Part model, mm, in its own coordinate system. A direction names the side the tool comes from. Round coordinates to 2 decimals unless told otherwise and drop trailing zeros. Write each loop counter-clockwise with the first axis right and the second up, starting at its lowest first coordinate (ties: lowest second). Pieces come first, ordered by that corner, then holes. Notation, with made-up numbers: M 21,0.25 L 61,0.25 A23 ccw 61,25.25 Z; hole C 36,-1 d2. An arc over 180 degrees is marked long. Use one line per item in the form item = value. Start each with the question number.
Item 1: Probe L1, parallel to X at y = 0, z = 15; L2, parallel to X at y = -1.5, z = 7.5; L3, parallel to Y at x = -19, z = 56. List the from-to ranges inside material, lowest first.
Item 2: Cut at A-A, the plane y = 0. Give the cut face in (x, z).
Item 3: Cut at D-D, the plane y = -5. Give the cut face in (x, z).
Item 4: Flat gauge pins, fed straight in: pin 1 Ø3 at (x, y) = (4, -20) entering from -Z; pin 2 Ø8 at (x, y) = (-16.46, 16.07) entering from +Z; pin 3 Ø1.5 at (x, z) = (5, 24.5) entering from -Y. Where does each tip first touch, or does it go through?
Item 5: Cut at B-B, the plane y = -14.5. Give the cut face in (x, z).
Item 6: Which spindle directions (+Z, -Z, +X, -X, +Y, -Y) get a long thin tool onto all of the face, cutting with end or side? Do faces 1 (the face through (0, 21, 56)), 2 (the face through (20.859, -21.297, 29.58)), 3 (the face through (-20, -2, 59)), 4 (the face through (0, -21, 52)), 5 (the face through (13.68, -18.2, 29.58)). Say none if no direction does.
Item 7: Cut at C-C, the plane z = 35.5. Give the cut face in (x, y), then the cut area to 3 significant figures.
Item 8: Mould opens along Z. For faces 6 (the face through (-28, 0, 30)), 7 (the face through (0, 21, 34)) say: +Z half, -Z half, draft (parallel to the pull), parting line (faces both ways), or undercut.
from build123d import *

# Parameters (mm, degrees)
SKETCH1_R               = 16
SKETCH1_R_2             = 3.5
SKETCH1_R_3             = 2
BOSS_EXTRUDE1_DEPTH     = 60
SKETCH2_R               = 18
SKETCH2_R_2             = 16
BOSS_EXTRUDE2_DEPTH     = 2
CUT_EXTRUDE1_DEPTH      = 2
SKETCH6_W               = 4
SKETCH6_H               = 24
LPATTERN1_COUNT         = 9
LPATTERN1_PITCH         = 6
MIRROR1_COPY_1_SKETCH_W = 4
MIRROR1_COPY_1_SKETCH_H = 24
MIRROR1_COPY_2_SKETCH_W = 4
MIRROR1_COPY_2_SKETCH_H = 24
MIRROR1_COPY_3_SKETCH_W = 4
MIRROR1_COPY_3_SKETCH_H = 24
MIRROR1_COPY_4_SKETCH_W = 4
MIRROR1_COPY_4_SKETCH_H = 24
MIRROR1_COPY_5_SKETCH_W = 4
MIRROR1_COPY_5_SKETCH_H = 24
MIRROR1_COPY_6_SKETCH_W = 4
MIRROR1_COPY_6_SKETCH_H = 24
MIRROR1_COPY_7_SKETCH_W = 4
MIRROR1_COPY_7_SKETCH_H = 24
MIRROR1_COPY_8_SKETCH_W = 4
MIRROR1_COPY_8_SKETCH_H = 24


with BuildPart() as part:
    # Sketch1 → Boss-Extrude1 (new body)
    with BuildSketch(Plane.XY):
        with BuildLine():
            Line((-24, 22.5), (18, 22.5))
            ThreePointArc((18, 22.5), (20.828427125, 21.328427125), (22, 18.5))
            Line((22, 18.5), (22, -18.5))
            ThreePointArc((22, -18.5), (20.828427125, -21.328427125), (18, -22.5))
            Line((18, -22.5), (-24, -22.5))
            ThreePointArc((-24, -22.5), (-26.828427125, -21.328427125), (-28, -18.5))
            Line((-28, -18.5), (-28, 18.5))
            ThreePointArc((-28, 18.5), (-26.828427125, 21.328427125), (-24, 22.5))
        make_face()
        Circle(SKETCH1_R, mode=Mode.SUBTRACT)
        with Locations((16.069433567, 16.455190818)):
            Circle(SKETCH1_R_2, mode=Mode.SUBTRACT)
        with Locations((16.455190818, -16.069433567)):
            Circle(SKETCH1_R_2, mode=Mode.SUBTRACT)
        with Locations((-16.069433567, -16.455190818)):
            Circle(SKETCH1_R_2, mode=Mode.SUBTRACT)
        with Locations((-16.455190818, 16.069433567)):
            Circle(SKETCH1_R_2, mode=Mode.SUBTRACT)
        with Locations((-24, 0)):
            Circle(SKETCH1_R_3, mode=Mode.SUBTRACT)
    extrude(amount=BOSS_EXTRUDE1_DEPTH)

    # Sketch2 → Boss-Extrude2 (add)
    with BuildSketch(Plane(origin=(0, 0, 0), x_dir=(-1, 0, 0), z_dir=(0, 0, -1))):
        Circle(SKETCH2_R)
        Circle(SKETCH2_R_2, mode=Mode.SUBTRACT)
    extrude(amount=BOSS_EXTRUDE2_DEPTH)

    # Sketch3 → Cut-Extrude1 (cut)
    with BuildSketch(Plane.XY.offset(60)):
        with BuildLine():
            Line((-24, -2), (-15.874507866, -2))
            ThreePointArc((-15.874507866, -2), (-16, 0), (-15.874507866, 2))
            Line((-15.874507866, 2), (-24, 2))
            ThreePointArc((-24, 2), (-22.585786438, 1.414213562), (-22, 0))
            ThreePointArc((-22, 0), (-22.585786438, -1.414213562), (-24, -2))
        make_face()
    extrude(amount=-CUT_EXTRUDE1_DEPTH, mode=Mode.SUBTRACT)

    # Sketch6 → Cut-Revolve1 (revolve, cut)
    with BuildSketch(Plane(origin=(0, 0, 0), x_dir=(0, 0, -1), z_dir=(1, 0, 0))):
        with Locations((-54, 30.5)):
            Rectangle(SKETCH6_W, SKETCH6_H)
    cut_revolve1 = revolve(axis=Axis((0, 42.5, 56), (0, 0, -1)), mode=Mode.SUBTRACT)

    # LPattern1: Cut-Revolve1 ×9
    with Locations(*[(0, 0, -i * LPATTERN1_PITCH) for i in range(1, LPATTERN1_COUNT)]):
        add(cut_revolve1, mode=Mode.SUBTRACT)

    # Mirror1: Cut-Revolve1 across plane
    add(cut_revolve1.mirror(Plane.ZX), mode=Mode.SUBTRACT)

    # Mirror1 copy 1 sketch → Mirror1 copy 1 (revolve, cut)
    with BuildSketch(Plane(origin=(0, 0, -6), x_dir=(0, 0, -1), z_dir=(1, 0, 0))):
        with Locations((-54, -30.5)):
            Rectangle(MIRROR1_COPY_1_SKETCH_W, MIRROR1_COPY_1_SKETCH_H)
    revolve(axis=Axis((0, -42.5, 50), (0, 0, 1)), mode=Mode.SUBTRACT)

    # Mirror1 copy 2 sketch → Mirror1 copy 2 (revolve, cut)
    with BuildSketch(Plane(origin=(0, 0, -12), x_dir=(0, 0, -1), z_dir=(1, 0, 0))):
        with Locations((-54, -30.5)):
            Rectangle(MIRROR1_COPY_2_SKETCH_W, MIRROR1_COPY_2_SKETCH_H)
    revolve(axis=Axis((0, -42.5, 44), (0, 0, 1)), mode=Mode.SUBTRACT)

    # Mirror1 copy 3 sketch → Mirror1 copy 3 (revolve, cut)
    with BuildSketch(Plane(origin=(0, 0, -18), x_dir=(0, 0, -1), z_dir=(1, 0, 0))):
        with Locations((-54, -30.5)):
            Rectangle(MIRROR1_COPY_3_SKETCH_W, MIRROR1_COPY_3_SKETCH_H)
    revolve(axis=Axis((0, -42.5, 38), (0, 0, 1)), mode=Mode.SUBTRACT)

    # Mirror1 copy 4 sketch → Mirror1 copy 4 (revolve, cut)
    with BuildSketch(Plane(origin=(0, 0, -24), x_dir=(0, 0, -1), z_dir=(1, 0, 0))):
        with Locations((-54, -30.5)):
            Rectangle(MIRROR1_COPY_4_SKETCH_W, MIRROR1_COPY_4_SKETCH_H)
    revolve(axis=Axis((0, -42.5, 32), (0, 0, 1)), mode=Mode.SUBTRACT)

    # Mirror1 copy 5 sketch → Mirror1 copy 5 (revolve, cut)
    with BuildSketch(Plane(origin=(0, 0, -30), x_dir=(0, 0, -1), z_dir=(1, 0, 0))):
        with Locations((-54, -30.5)):
            Rectangle(MIRROR1_COPY_5_SKETCH_W, MIRROR1_COPY_5_SKETCH_H)
    revolve(axis=Axis((0, -42.5, 26), (0, 0, 1)), mode=Mode.SUBTRACT)

    # Mirror1 copy 6 sketch → Mirror1 copy 6 (revolve, cut)
    with BuildSketch(Plane(origin=(0, 0, -36), x_dir=(0, 0, -1), z_dir=(1, 0, 0))):
        with Locations((-54, -30.5)):
            Rectangle(MIRROR1_COPY_6_SKETCH_W, MIRROR1_COPY_6_SKETCH_H)
    revolve(axis=Axis((0, -42.5, 20), (0, 0, 1)), mode=Mode.SUBTRACT)

    # Mirror1 copy 7 sketch → Mirror1 copy 7 (revolve, cut)
    with BuildSketch(Plane(origin=(0, 0, -42), x_dir=(0, 0, -1), z_dir=(1, 0, 0))):
        with Locations((-54, -30.5)):
            Rectangle(MIRROR1_COPY_7_SKETCH_W, MIRROR1_COPY_7_SKETCH_H)
    revolve(axis=Axis((0, -42.5, 14), (0, 0, 1)), mode=Mode.SUBTRACT)

    # Mirror1 copy 8 sketch → Mirror1 copy 8 (revolve, cut)
    with BuildSketch(Plane(origin=(0, 0, -48), x_dir=(0, 0, -1), z_dir=(1, 0, 0))):
        with Locations((-54, -30.5)):
            Rectangle(MIRROR1_COPY_8_SKETCH_W, MIRROR1_COPY_8_SKETCH_H)
    revolve(axis=Axis((0, -42.5, 8), (0, 0, 1)), mode=Mode.SUBTRACT)


solid = part.part
Model answer:
q1.L1 = -28 to -26, -22 to -16, 16 to 22
q1.L2 = -28 to -25.32, -22.68 to -15.93, 15.93 to 22
q1.L3 = -22.5 to -18.37, -14.54 to 13.67, 18.47 to 22.5
q2.outline = M -28,0 L -26,0 L -26,60 L -28,60 Z; M -22,0 L -18,0 L -18,-2 L -16,-2 L -16,58 L -22,58 Z; M 16,-2 L 18,-2 L 18,0 L 22,0 L 22,60 L 16,60 Z
q3.outline = M -28,0 L -17.29,0 L -17.29,-2 L -15.2,-2 L -15.2,60 L -28,60 Z; M 15.2,-2 L 17.29,-2 L 17.29,0 L 22,0 L 22,60 L 15.2,60 Z
q4.pin_1 = 0
q4.pin_2 = 60
q4.pin_3 = -19.2
q5.outline = M -28,0 L -18.97,0 L -18.97,60 L -28,60 Z; M -13.17,0 L -10.67,0 L -10.67,-2 L -6.76,-2 L -6.76,60 L -13.17,60 Z; M 6.76,-2 L 10.67,-2 L 10.67,0 L 13.33,0 L 13.33,60 L 6.76,60 Z; M 19.58,0 L 22,0 L 22,60 L 19.58,60 Z
q6.face_1 = +Y
q6.face_2 = +Z, -Z, +X, -Y
q6.face_3 = +Z
q6.face_4 = -Y
q6.face_5 = +Z, -Z
q7.outline = M -28,-18.5 A4 ccw -24,-22.5 L -13.27,-22.5 A24 cw 13.27,-22.5 L 18,-22.5 A4 ccw 22,-18.5 L 22,18.5 A4 ccw 18,22.5 L 13.27,22.5 A24 cw -13.27,22.5 L -24,22.5 A4 ccw -28,18.5 Z; hole C -24,0 d4; hole C -16.46,16.07 d7; hole C -16.07,-16.46 d7; hole C 0,0 d32; hole C 16.07,16.46 d7; hole C 16.46,-16.07 d7
q7.area = 1,120 mm²
q8.face_6 = draft
q8.face_7 = undercut
